from build123d import *

# Parameters (mm, degrees)
SKETCH2_W           = 63.5
SKETCH2_H           = 44.45
BOSS_EXTRUDE1_DEPTH = 25.4
SKETCH3_W           = 63.5
SKETCH3_H           = 12.2
CUT_EXTRUDE1_DEPTH  = 3.048
SKETCH4_R           = 1.6
CUT_EXTRUDE2_DEPTH  = 47.337599474
SKETCH10_R          = 1.5875
CUT_EXTRUDE3_DEPTH  = 6.35
SKETCH8_R           = 1.5875
CUT_EXTRUDE4_DEPTH  = 6.35
SKETCH5_R           = 1.5875
CUT_EXTRUDE5_DEPTH  = 6.35
SKETCH6_R           = 1.5875
CUT_EXTRUDE6_DEPTH  = 6.35
SKETCH11_W          = 39.6875
SKETCH11_H          = 15.875
CUT_EXTRUDE8_DEPTH  = 1.5875


with BuildPart() as part:
    # Sketch2 → Boss-Extrude1 (new body)
    with BuildSketch(Plane(origin=(0, 0, 0), x_dir=(1, 0, 0), z_dir=(0, 1, 0))):
        Rectangle(SKETCH2_W, SKETCH2_H)
    extrude(amount=BOSS_EXTRUDE1_DEPTH)

    # Sketch3 → Cut-Extrude1 (cut)
    with BuildSketch(Plane.XZ):
        Rectangle(SKETCH3_W, SKETCH3_H)
    extrude(amount=-CUT_EXTRUDE1_DEPTH, mode=Mode.SUBTRACT)

    # Sketch4 → Cut-Extrude2 (cut, through all)
    with BuildSketch(Plane(origin=(0, 25.4, 0), x_dir=(1, 0, 0), z_dir=(0, 1, 0))):
        with Locations(Location((-12.5, 0, 0), (0, 0, 270))):
            Circle(SKETCH4_R)
        with Locations(Location((12.5, 0, 0), (0, 0, 270))):
            Circle(SKETCH4_R)
    extrude(amount=-CUT_EXTRUDE2_DEPTH, mode=Mode.SUBTRACT)

    # Sketch10 → Cut-Extrude3 (cut)
    with BuildSketch(Plane(origin=(31.75, 0, 0), x_dir=(0, 0, -1), z_dir=(1, 0, 0))):
        with Locations((15.875, 20.590962003)):
            Circle(SKETCH10_R)
    extrude(amount=-CUT_EXTRUDE3_DEPTH, mode=Mode.SUBTRACT)

    # Sketch8 → Cut-Extrude4 (cut)
    with BuildSketch(Plane(origin=(31.75, 1.540962003, -6.057895699), x_dir=(0, 0, -1), z_dir=(1, 0, 0))):
        with Locations((-10.820395699, 19.05)):
            Circle(SKETCH8_R)
    extrude(amount=-CUT_EXTRUDE4_DEPTH, mode=Mode.SUBTRACT)

    # Sketch5 → Cut-Extrude5 (cut)
    with BuildSketch(Plane(origin=(31.75, 1.540962003, -6.057895699), x_dir=(0, 0, -1), z_dir=(1, 0, 0))):
        with Locations((-23.520395699, 19.05)):
            Circle(SKETCH5_R)
    extrude(amount=-CUT_EXTRUDE5_DEPTH, mode=Mode.SUBTRACT)

    # Sketch6 → Cut-Extrude6 (cut)
    with BuildSketch(Plane(origin=(31.75, 1.540962003, -6.057895699), x_dir=(0, 0, -1), z_dir=(1, 0, 0))):
        with Locations((-23.520395699, 9.525)):
            Circle(SKETCH6_R)
    extrude(amount=-CUT_EXTRUDE6_DEPTH, mode=Mode.SUBTRACT)

    # Sketch11 → Cut-Extrude8 (cut)
    with BuildSketch(Plane(origin=(31.75, 1.540962003, -6.057895699), x_dir=(0, 0, -1), z_dir=(1, 0, 0))):
        with Locations((-6.851645699, 14.2875)):
            Rectangle(SKETCH11_W, SKETCH11_H)
    extrude(amount=-CUT_EXTRUDE8_DEPTH, mode=Mode.SUBTRACT)


solid = part.part
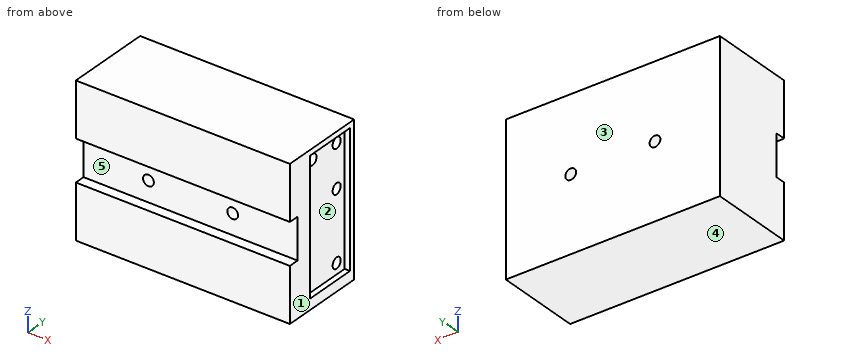
Design review of the part built by this model. Coordinates are the model's own, in mm. Face numbers are marked on the shaded views. A direction names the side the tool comes from. Give positions to 0.01 mm unless a question says otherwise; leave off trailing zeros. Order: outer loops, then holes, each group sorted by start corner. A loop starts at its lowest first (then second) coordinate and runs counter-clockwise, first axis right, second up. Notation, with made-up numbers: (28.5, 1.5) - (46.5, 1.5) arc R9 ccw to (46.5, 13.5) - close; hole circle Ø1 at (-17, 19.5). An arc over 180 degrees is marked (long way). Write item = value, one per line. Start each with the question number.
Q1. To check wall thickness, follow L1, parallel to X at y = 19.25, z = 0; L2, parallel to Z at x = -12.5, y = 1.75 (3 decimals); L3, parallel to Y at x = -21.5, z = 3. State the ranges of each line that lie inside material, in increasing order. Write a range as from..to.
Q2. Tool access review of the marked faces 1 and 2: name each direction out of +Z, -Z, +X, -X, +Y, -Y from which nothing blocks a thin tool from reaching the whole face with its end or side.
Q3. We need section B-B on z = 0. State the section outline as (x, y) points, plus the area to 3 significant figures.
Q4. Mouldability with a two-part tool opening along Z and no side actions: class the marked faces 3, 4 and 5 as released by +Z, released by -Z, zero draft, split by the parting line, or undercut.
Q5. Clearance check with flat-ended pins moving along their axes: pin 1 Ø6 at (x, z) = (-16, -2.5) entering from -Y; pin 2 Ø1.6 at (y, z) = (21, -16) entering from +X; pin 3 Ø4 at (x, z) = (-22, 6) entering from -Y; pin 4 Ø2.5 at (y, z) = (11.5, 18) entering from +X. State where each tip first meets the part, or that it passes through.
Q6. We need section C-C on y = 13.75. State how many separate pieces and enclosed holes the cut face has, plus the area to 3 significant figures.
Q7. We need section D-D on z = -8. State the section outline as (x, y) points, plus the area to 3 significant figures.
Q8. We need section A-A on x = 12.5. State the section outline as (y, z) points (3 decimals), plus the area to 3 significant figures.
Working result:
q1.L1 = -31.75..-14.1, -10.9..10.9, 14.1..30.16
q1.L2 = -22.225..-6.1, 6.1..22.225
q1.L3 = 3.05..25.4
q2.face_1 = +Z, -Z, +X, +Y, -Y
q2.face_2 = +X
q3.outline = (-31.75, 3.05) - (-14.1, 3.05) - (-14.1, 25.4) - (-31.75, 25.4) - close; (-10.9, 3.05) - (10.9, 3.05) - (10.9, 25.4) - (-10.9, 25.4) - close; (14.1, 3.05) - (31.75, 3.05) - (31.75, 7.89) - (30.16, 7.89) - (30.16, 23.77) - (31.75, 23.77) - (31.75, 25.4) - (14.1, 25.4) - close
q3.area = 1,250 mm²
q4.face_3 = zero draft
q4.face_4 = released by -Z
q4.face_5 = undercut
q5.pin_1 = 3.05
q5.pin_2 = 25.4
q5.pin_3 = 0
q5.pin_4 = 30.16
q6.separate_pieces = 1
q6.enclosed_holes = 2
q6.area = 2,740 mm²
q7.outline = (-31.75, 0) - (31.75, 0) - (31.75, 7.89) - (30.16, 7.89) - (30.16, 23.77) - (31.75, 23.77) - (31.75, 25.4) - (-31.75, 25.4) - close
q7.area = 1,590 mm²
q8.outline = (0, -22.225) - (25.4, -22.225) - (25.4, -1.6) - (3.048, -1.6) - (3.048, -6.1) - (0, -6.1) - close; (0, 6.1) - (3.048, 6.1) - (3.048, 1.6) - (25.4, 1.6) - (25.4, 22.225) - (0, 22.225) - close
q8.area = 1,020 mm²
